Check sheet for the modelled part. Datum: model origin and axes. Units: mm. A direction names the side the tool comes from. Coordinates: 2 decimals unless noted, no trailing zeros. Order: outer loops, then holes, each group sorted by start corner. A loop starts at its lowest first (then second) coordinate and runs counter-clockwise, first axis right, second up.
1. Draft check along X on faces 3 (the flat face through (-94, -15, 36.636)), 4 (the flat face through (-212, -30, 7)), 5 (the flat face through (57.758, -19, 7)), 6 (the cylindrical face through (50.236, -14.79, 7.625)). Enter one of: released by +X, released by -X, zero draft, split by the parting line, or undercut.
2. Gauge pin test, flat ends, axial feed: pin 1 Ø3 at (x, z) = (-47.5, 24) entering from -Y; pin 2 Ø13.5 at (x, z) = (-86.5, 15) entering from +Y; pin 3 Ø8 at (x, z) = (-203.5, 24.5) entering from +Y; pin 4 Ø3 at (y, z) = (-35, 27.5) entering from +X. Record the tip position at first contact, or that the pin passes through.
3. Cross-section at B-B (x = -48). Enter the section's corners in (y, z), then the cut area to 3 significant figures.
4. Cross-section at A-A (y = -16). Enter the section's corners in (x, z), then the cut area to 3 significant figures.
5. Set-up check for faces 1 (the flat face through (-94.34, -40.14, 6.22)), 2 (the flat face through (28, -30, 7)): record each of +Z, -Z, +X, -X, +Y, -Y from which the full face is reachable in a straight line by a thin tool's end or side.
6. Cross-section at C-C (z = 26). Enter the section's corners in (x, y).
7. Thickness scan on line 1 (X direction, y = -21, z = 21); line 2 (X direction, y = -6.5, z = -10.5); line 3 (Z direction, x = -208, y = -3). Record the ranges inside material, lowest first.
8. Cross-section at D-D (x = -5). Enter the section's corners in (y, z).
```python
from build123d import *

# Parameters (mm, degrees)
F0_W     = 300
F0_H     = 60
F1_DEPTH = 30
F3_DEPTH = 300
F4_R     = 22.5
F5_DEPTH = 30


with BuildPart() as f1:
    # F0 (on Front) → F1 (new body)
    with BuildSketch(Plane.XZ):
        with Locations((-92.24209, 6.635918)):
            Rectangle(F0_W, F0_H)
    extrude(amount=F1_DEPTH)

    # F2 (on face) → F3 (join)
    with BuildSketch(Plane(origin=(-242.24209, 0, 0), x_dir=(0, -1, 0), z_dir=(-1, 0, 0))):
        Polygon((30, 36.635918), (30, -23.364082), (50, -23.364082), align=None)
    extrude(amount=-F3_DEPTH)

    # F4 (on face) → F5 (cut)
    with BuildSketch(Plane(origin=(0, 0, 0), x_dir=(-1, 0, 0), z_dir=(0, 1, 0))):
        with Locations((-27.75791, 6.635918)):
            Circle(F4_R)
        with BuildLine():
            ThreePointArc((54.74209, 6.635918), (48.151992, 22.545821), (32.24209, 29.135918))
            ThreePointArc((32.24209, 29.135918), (16.332187, -9.273985), (54.74209, 6.635918))
        make_face()
        with BuildLine():
            ThreePointArc((114.74209, 6.635918), (108.151992, 22.545821), (92.24209, 29.135918))
            ThreePointArc((92.24209, 29.135918), (76.332187, -9.273985), (114.74209, 6.635918))
        make_face()
        with BuildLine():
            ThreePointArc((174.74209, 6.635918), (168.151992, 22.545821), (152.24209, 29.135918))
            ThreePointArc((152.24209, 29.135918), (136.332187, -9.273985), (174.74209, 6.635918))
        make_face()
        with Locations((212.24209, 6.635918)):
            Circle(F4_R)
    extrude(amount=-F5_DEPTH, mode=Mode.SUBTRACT)


solid = f1.part
```
Data:
1. face 3: zero draft
1. face 4: undercut
1. face 5: released by +X
1. face 6: undercut
2. pin 1: stops at y = -34.71
2. pin 2: stops at y = -30
2. pin 3: stops at y = 0
2. pin 4: passes through
3. outline: (-50, -23.36) - (0, -23.36) - (0, -9.42) - (-30, -9.42) - (-30, 22.7) - (0, 22.7) - (0, 36.64) - (-30, 36.64) - close
3. area: 1,440 mm2
4. outline: (-242.24, -23.36) - (57.76, -23.36) - (57.76, 36.64) - (-242.24, 36.64) - close; hole circle Ø45 at (-212.24, 6.64); hole circle Ø45 at (-152.24, 6.64); hole circle Ø45 at (-92.24, 6.64); hole circle Ø45 at (-32.24, 6.64); hole circle Ø45 at (27.76, 6.64)
4. area: 10,000 mm2
5. face 1: +Z, +X, -X, -Y
5. face 2: +Y
6. outline: (-242.24, -33.55) - (57.76, -33.55) - (57.76, 0) - (39.22, 0) - (39.22, -30) - (16.3, -30) - (16.3, 0) - (-20.78, 0) - (-20.78, -30) - (-43.7, -30) - (-43.7, 0) - (-80.78, 0) - (-80.78, -30) - (-103.7, -30) - (-103.7, 0) - (-140.78, 0) - (-140.78, -30) - (-163.7, -30) - (-163.7, 0) - (-200.78, 0) - (-200.78, -30) - (-223.7, -30) - (-223.7, 0) - (-242.24, 0) - close
7. line 1: x = -242.24 to -229.56, -194.92 to -169.56, -134.92 to -109.56, -74.92 to -49.56, -14.92 to 10.44, 45.08 to 57.76
7. line 2: x = -242.24 to -226.82, -197.66 to -166.82, -137.66 to -106.82, -77.66 to -46.82, -17.66 to 13.18, 42.34 to 57.76
7. line 3: z = -23.36 to -15.46, 28.73 to 36.64
8. outline: (-50, -23.36) - (0, -23.36) - (0, 36.64) - (-30, 36.64) - close
